from build123d import *

# Parameters (mm, degrees)
SKETCH1_W           = 14.25
SKETCH1_H           = 29
SKETCH1_R           = 1.375
BOSS_EXTRUDE1_DEPTH = 1.5
SKETCH2_W           = 12.5
SKETCH2_H           = 16
BOSS_EXTRUDE2_DEPTH = 5.5
SKETCH4_R           = 0.375
LPATTERN1_COUNT     = 2
LPATTERN1_PITCH     = 2.54
LPATTERN1_COL_COUNT = 2
LPATTERN1_COL_PITCH = 2.54
MOVE_FACE1_BY       = 8.2
MOVE_FACE1_2_BY     = 8.2
MOVE_FACE1_3_BY     = 8.2


with BuildPart() as part:
    # Sketch1 → Boss-Extrude1 (new body)
    with BuildSketch(Plane(origin=(0, 0, 0), x_dir=(1, 0, 0), z_dir=(0, 1, 0))):
        Rectangle(SKETCH1_W, SKETCH1_H)
        with Locations(Location((0, -8.025, 0), (0, 0, 270))):
            Circle(SKETCH1_R, mode=Mode.SUBTRACT)
    extrude(amount=BOSS_EXTRUDE1_DEPTH)

    # Sketch2 → Boss-Extrude2 (add)
    with BuildSketch(Plane(origin=(0, 1.5, 0), x_dir=(1, 0, 0), z_dir=(0, 1, 0))):
        with Locations((0, 6.5)):
            Rectangle(SKETCH2_W, SKETCH2_H)
    extrude(amount=BOSS_EXTRUDE2_DEPTH)

    # Sweep1: sweep along a path in Sketch3
    with BuildLine(Plane.ZY) as sweep1_path:
        Line((13.5, -1), (13.5, 5.5))
        ThreePointArc((13.5, 5.5), (13.792893219, 6.207106781), (14.5, 6.5))
        Line((14.5, 6.5), (20.8, 6.5))
    # Sketch4 → Sweep1 (sweep)
    with BuildSketch(Plane(origin=(0, -1, 0), x_dir=(-1, 0, 0), z_dir=(0, -1, 0))):
        with Locations((0, -13.5)):
            Circle(SKETCH4_R)
    sweep1 = sweep(path=sweep1_path.line)

    # LPattern1: Sweep1 ×2
    with Locations(*[(-i * LPATTERN1_PITCH, 0, 0) for i in range(1, LPATTERN1_COUNT)]):
        add(sweep1)

    # LPattern1 col: Sweep1 ×2
    with Locations(*[(i * LPATTERN1_COL_PITCH, 0, 0) for i in range(1, LPATTERN1_COL_COUNT)]):
        add(sweep1)

    # Move Face1: a face moved outward by 8.2
    extrude(part.faces().sort_by_distance((2.54, -1, 13.5))[0], amount=MOVE_FACE1_BY, dir=(0, -1, 0))

    # Move Face1 2: a face moved outward by 8.2
    extrude(part.faces().sort_by_distance((0, -1, 13.5))[0], amount=MOVE_FACE1_2_BY, dir=(0, -1, 0))

    # Move Face1 3: a face moved outward by 8.2
    extrude(part.faces().sort_by_distance((-2.54, -1, 13.5))[0], amount=MOVE_FACE1_3_BY, dir=(0, -1, 0))


solid = part.part
The listing builds one solid part. Answer for the finished solid, in the listing's coordinates (mm). A direction names the side the tool comes from. Round coordinates to 2 decimals unless told otherwise and drop trailing zeros. Write each loop counter-clockwise with the first axis right and the second up, starting at its lowest first coordinate (ties: lowest second). Pieces come first, ordered by that corner, then holes. Notation, with made-up numbers: M -11.5,42 L 26.5,42 A22 ccw 26.5,71 Z; hole C 22.5,-10.5 d9. An arc over 180 degrees is marked long. Write each question's results on one line, items separated by ' | '. Start each with the question number.
Item 1: Straight lines are drawn through the part: L1, parallel to Y at x = 5, z = 3; L2, parallel to Z at x = -6, y = 0.5; L3, parallel to Z at x = -5.5, y = 4.5. For each, find the intervals that lie inside material, in ascending order. Write a range as [from, to].
Item 2: A cutting plane is placed at C-C on x = -2.54. Write down the section's boundary in (y, z) (3 decimals).
Item 3: A cutting plane is placed at A-A on x = 0. Write down the section's boundary in (y, z) (3 decimals).
Item 4: For a pull along Z with two mould halves and no side action, classify faces 1 (the face through (0, 4, 1.5)), 2 (the face through (0.06, 0.74, 6.65)), 3 (the face through (6.25, 4, -6)), 4 (the face through (0, 3, -14.5)) as pulls with the +Z half, pulls with the -Z half, needs draft (parallel to the pull), parting line crosses it, or undercut.
Item 5: A cutting plane is placed at D-D on z = -3. Write down the section's boundary in (x, y) (3 decimals), and give its area (3 significant figures).
Item 6: A cutting plane is placed at B-B on y = 3.75. Write down the section's boundary in (x, z) (3 decimals).
Item 7: Flat-ended cylindrical pins translate along their axes: pin 1 Ø4.5 at (x, z) = (-3, 2) entering from +Y; pin 2 Ø6 at (x, y) = (-1, -5.5) entering from -Z (3 decimals); pin 3 Ø3 at (y, z) = (4, -5.5) entering from -X; pin 4 Ø5 at (x, y) = (-5.5, -5) entering from -Z. Find the tip coordinate at first contact, or state that the pin passes through.
Item 8: For faces 5 (the face through (-6.25, 4, -6)), 6 (the face through (7.125, 1, 0)), determine the directions among +Z, -Z, +X, -X, +Y, -Y from which every point of the face is accessible in a straight line to the end or side of a thin tool.
Check sheet entries:
1) L1: [0, 1.5] | L2: [-14.5, 14.5] | L3: [-14.5, 1.5]
2) outline: M -9.2,13.125 L 0,13.125 L 0,-14.5 L 7,-14.5 L 7,1.5 L 1.5,1.5 L 1.5,13.125 L 5.5,13.125 A1.375 ccw 6.875,14.5 L 6.875,20.8 L 6.125,20.8 L 6.125,14.5 A0.625 cw 5.5,13.875 L 1.5,13.875 L 1.5,14.5 L 0,14.5 L 0,13.875 L -9.2,13.875 Z
3) outline: M -9.2,13.125 L 0,13.125 L 0,9.4 L 1.5,9.4 L 1.5,13.125 L 5.5,13.125 A1.375 ccw 6.875,14.5 L 6.875,20.8 L 6.125,20.8 L 6.125,14.5 A0.625 cw 5.5,13.875 L 1.5,13.875 L 1.5,14.5 L 0,14.5 L 0,13.875 L -9.2,13.875 Z; M 0,-14.5 L 7,-14.5 L 7,1.5 L 1.5,1.5 L 1.5,6.65 L 0,6.65 Z
4) face 1: undercut | face 2: undercut | face 3: needs draft | face 4: pulls with the -Z half
5) outline: M -7.125,0 L 7.125,0 L 7.125,1.5 L 6.25,1.5 L 6.25,7 L -6.25,7 L -6.25,1.5 L -7.125,1.5 Z | area: 90.1 mm²
6) outline: M -6.25,-14.5 L 6.25,-14.5 L 6.25,1.5 L -6.25,1.5 Z; C -2.54,13.5 d0.75; C 0,13.5 d0.75; C 2.54,13.5 d0.75
7) pin 1: y = 7 | pin 2: z = 13.125 | pin 3: x = -6.25 | pin 4: through
8) face 5: +Z, -Z, -X, +Y | face 6: +Z, -Z, +X, +Y, -Y
